```python
from build123d import *

# Parameters (mm, degrees)
MODEL_R             = 1.5
MODEL_R_2           = 5
MODEL_R_3           = 6
BOSS_EXTRUDE1_DEPTH = 2


with BuildPart() as part:
    # Model → Boss-Extrude1 (new body)
    with BuildSketch(Plane.XY):
        with BuildLine():
            Line((-87.5, 25), (87.5, 25))
            ThreePointArc((87.5, 25), (89.267766953, 24.267766953), (90, 22.5))
            Line((90, 22.5), (90, 2.5))
            ThreePointArc((90, 2.5), (89.267766953, 0.732233047), (87.5, 0))
            Line((87.5, 0), (-87.5, 0))
            ThreePointArc((-87.5, 0), (-89.267766953, 0.732233047), (-90, 2.5))
            Line((-90, 2.5), (-90, 22.5))
            ThreePointArc((-90, 22.5), (-89.267766953, 24.267766953), (-87.5, 25))
        make_face()
        with Locations((86, 12.5)):
            Circle(MODEL_R, mode=Mode.SUBTRACT)
        with Locations(Location((-86, 12.5, 0), (0, 0, 180))):
            Circle(MODEL_R, mode=Mode.SUBTRACT)
        with Locations((0, 12.5)):
            Circle(MODEL_R_2, mode=Mode.SUBTRACT)
        with Locations((-70, 12.5)):
            Circle(MODEL_R_3, mode=Mode.SUBTRACT)
        with Locations(Location((70, 12.5, 0), (0, 0, 180))):
            Circle(MODEL_R_3, mode=Mode.SUBTRACT)
        with Locations((-54, 12.5)):
            Circle(MODEL_R, mode=Mode.SUBTRACT)
        with Locations(Location((54, 12.5, 0), (0, 0, 180))):
            Circle(MODEL_R, mode=Mode.SUBTRACT)
        with Locations((-30, 12.5)):
            Circle(MODEL_R, mode=Mode.SUBTRACT)
        with Locations(Location((30, 12.5, 0), (0, 0, 180))):
            Circle(MODEL_R, mode=Mode.SUBTRACT)
    extrude(amount=BOSS_EXTRUDE1_DEPTH)


solid = part.part
```
Part model, mm, in its own coordinate system. Round coordinates to 2 decimals unless told otherwise and drop trailing zeros. Write each loop counter-clockwise with the first axis right and the second up, starting at its lowest first coordinate (ties: lowest second). Pieces come first, ordered by that corner, then holes.
Item 1: Probe L1, parallel to Y at x = -30, z = 1.5; L2, parallel to X at y = 7, z = 1.75; L3, parallel to Y at x = -70, z = 1.55. List the from-to ranges inside material, lowest first.
Results:
L1: y = 0 to 11, 14 to 25
L2: x = -90 to -72.4, -67.6 to 67.6, 72.4 to 90
L3: y = 0 to 6.5, 18.5 to 25
Item 2: Two-plate mould, pull along X, no slides. Class faces 1 (the flat face through (1, 18, 2)), 2 (the cylindrical face through (55.2, 13.4, 1)): +X half, -X half, draft (parallel to the pull), parting line (faces both ways), or undercut.
Results:
face 1: draft
face 2: undercut
Item 3: Cut at A-A, the plane x = 86. Give the cut face in (y, z).
Results:
outline: (0, 0) - (11, 0) - (11, 2) - (0, 2) - close; (14, 0) - (25, 0) - (25, 2) - (14, 2) - close
Item 4: Cut at B-B, the plane z = 0.35. Count the separate pieces of the cut face and the enclosed holes in it, plus the area to 3 significant figures.
Results:
separate pieces: 1
enclosed holes: 9
area: 4,150 mm2
Item 5: Drop a flat-ended pin along its axis: pin 1 Ø2.5 at (x, y) = (-30, 12.5) entering from -Z. Give the stop position or say it passes through.
Results:
pin 1: passes through
